Geometry check sheet. Reference: the model listing, model coordinates, mm. A direction names the side the tool comes from. Give positions to 0.01 mm unless a question says otherwise; leave off trailing zeros. Order: outer loops, then holes, each group sorted by start corner. A loop starts at its lowest first (then second) coordinate and runs counter-clockwise, first axis right, second up. Notation, with made-up numbers: M 31.25,4 L 89.25,4 A30 ccw 89.25,33 Z; hole C 2.5,79.25 d7. An arc over 180 degrees is marked long. Answer as CSV lines item,"result". Start each with the question number.
Q1. Mould release check, pull along X, two halves, no side actions. Record for faces 1 (the flat face through (22, 25, 5)), 2 (the flat face through (8.123, 7.007, 2.792)), 3 (the flat face through (13.75, 4, 3)), 4 (the flat face through (11, 1, 4)): +X half, -X half, draft (parallel to the pull), parting line (faces both ways), or undercut.
Q2. Set-up check for faces 5 (the flat face through (18.715, 24.992, 11.067)), 6 (the flat face through (11, 5, 1.55)): record each of +Z, -Z, +X, -X, +Y, -Y from which the full face is reachable in a straight line by a thin tool's end or side.
Q3. Section check C-C, the plane y = 6. Record the boundary of the cut face in (x, z).
Q4. Section check D-D, the plane z = 8. Record the boundary of the cut face in (x, y).
Q5. Section check B-B, the plane z = 3. Record the boundary of the cut face in (x, y).
Q6. Thickness scan on line 1 (X direction, y = 29, z = 11.5); line 2 (Z direction, x = 20.5, y = 2.5); line 3 (Z direction, x = 8, y = 29). Record the ranges inside material, lowest first.
Q7. Go/stop test with flat-tipped pins: pin 1 (1 mm diameter, centred on x = 6.5, z = 9, fed in from -Y); pin 2 (6.5 mm diameter, centred on x = 11, y = 5.5, fed in from +Z); pin 3 (4 mm diameter, centred on x = 18.5, y = 15, fed in from +Z). Record where each tip stops, or that it passes through.
Q8. Section check A-A, the plane x = 13. Record the boundary of the cut face in (y, z).
```python
from build123d import *

# Parameters (mm, degrees)
F0_W      = 22
F0_H      = 42
F1_DEPTH  = 4
F3_DEPTH  = 2.45
F5_DEPTH  = 3.8
F7_DEPTH  = 9.04
F9_DEPTH  = 6.48
F11_DEPTH = 6.48


with BuildPart() as f1:
    # F0 (on Top) → F1 (new body)
    with BuildSketch(Plane.XY):
        with Locations((11, 21)):
            Rectangle(F0_W, F0_H)
    extrude(amount=F1_DEPTH)

    # F2 (on face) → F3 (cut)
    with BuildSketch(Plane.XY.offset(4)):
        Polygon((8.25, 6.5), (8.25, 1.5), (13.75, 1.5), (13.75, 6.5), (14, 7.5), (8, 7.5), align=None)
    extrude(amount=-F3_DEPTH, mode=Mode.SUBTRACT)

    # F4 (on face) → F5 (cut)
    with BuildSketch(Plane.XY.offset(4)):
        Polygon((8, 7.5), (11, 7.5), (14, 7.5), (15.52, 7.5), (15.52, 42), (6.48, 42), (6.48, 7.5), align=None)
    extrude(amount=-F5_DEPTH, mode=Mode.SUBTRACT)

    # F6 (on face) → F7 (join)
    with BuildSketch(Plane.YZ.offset(6.48)):
        Polygon((42, 14.138905), (16.90533, 4), (42, 4), align=None)
        Polygon((16.90533, 4), (7.5, 0.2), (36.424737, 0.2), (42, 0.2), (42, 4), align=None)
    extrude(amount=F7_DEPTH)

    # F8 (on face) → F9 (join)
    with BuildSketch(Plane.YZ.offset(15.52)):
        Polygon((16.90533, 4), (42, 14.138905), (42, 17.938905), (7.5, 4), align=None)
        Polygon((42, 4), (42, 14.138905), (16.90533, 4), align=None)
    extrude(amount=F9_DEPTH)

    # F10 (on face) → F11 (join)
    with BuildSketch(Plane(origin=(6.48, 0, 0), x_dir=(0, -1, 0), z_dir=(-1, 0, 0))):
        Polygon((-42, 17.938905), (-42, 14.138905), (-16.90533, 4), (-7.5, 4), align=None)
        Polygon((-16.90533, 4), (-42, 14.138905), (-42, 4), align=None)
    extrude(amount=F11_DEPTH)


solid = f1.part
```
Answer block:
1,face 1,"+X half"
1,face 2,"undercut"
1,face 3,"undercut"
1,face 4,"draft"
2,face 5,"+Z, +X, -X, -Y"
2,face 6,"+Z"
3,outline,"M 0,0 L 22,0 L 22,4 L 13.75,4 L 13.75,1.55 L 8.25,1.55 L 8.25,4 L 0,4 Z"
4,outline,"M 0,17.4 L 6.48,17.4 L 6.48,26.81 L 15.52,26.81 L 15.52,17.4 L 22,17.4 L 22,42 L 0,42 Z"
5,outline,"M 0,0 L 22,0 L 22,42 L 0,42 Z; hole M 6.48,7.5 L 8,7.5 L 8.25,6.5 L 8.25,1.5 L 13.75,1.5 L 13.75,6.5 L 14,7.5 L 15.52,7.5 L 15.52,14.43 L 6.48,14.43 Z"
6,line 1,"x = 0 to 6.48, 15.52 to 22"
6,line 2,"z = 0 to 4"
6,line 3,"z = 0 to 8.89"
7,pin 1,"stops at y = 18.64"
7,pin 2,"stops at z = 4"
7,pin 3,"stops at z = 7.84"
8,outline,"M 0,0 L 42,0 L 42,14.14 L 7.5,0.2 L 7.5,1.55 L 1.5,1.55 L 1.5,4 L 0,4 Z"
